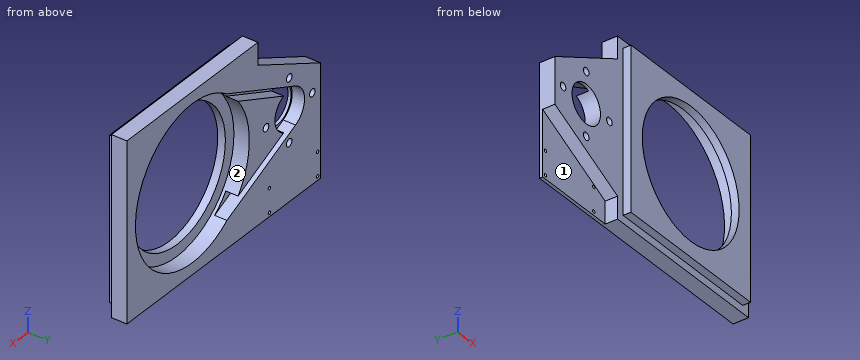
```python
from build123d import *

# Parameters (mm, degrees)
SKETCH1_W             = 105
SKETCH1_H             = 105
BOSS_EXTRUDE1_DEPTH   = 5
SKETCH2_W             = 115
SKETCH2_H             = 115
BOSS_EXTRUDE2_DEPTH   = 10
SKETCH3_R             = 42.5
CUT_EXTRUDE1_DEPTH    = 83.689177043
SKETCH4_R             = 50
CUT_EXTRUDE2_DEPTH    = 10
BOSS_EXTRUDE3_DEPTH   = 10
SKETCH6_R             = 12.5
CUT_EXTRUDE3_DEPTH    = 128.2301065
F_8_CLEARANCE_HOLE1_D = 4.9149
CUT_EXTRUDE4_DEPTH    = 8
SKETCH10_R            = 1
BOSS_EXTRUDE4_DEPTH   = 2


with BuildPart() as part:
    # Sketch1 → Boss-Extrude1 (new body)
    with BuildSketch(Plane(origin=(0, 0, 0), x_dir=(1, 0, 0), z_dir=(0, 1, 0))):
        Rectangle(SKETCH1_W, SKETCH1_H)
    extrude(amount=BOSS_EXTRUDE1_DEPTH)

    # Sketch2 → Boss-Extrude2 (add)
    with BuildSketch(Plane(origin=(0, 5, 0), x_dir=(1, 0, 0), z_dir=(0, 1, 0))):
        Rectangle(SKETCH2_W, SKETCH2_H)
    extrude(amount=BOSS_EXTRUDE2_DEPTH)

    # Sketch3 → Cut-Extrude1 (cut, through all)
    with BuildSketch(Plane(origin=(0, 15, 0), x_dir=(1, 0, 0), z_dir=(0, 1, 0))):
        with Locations(Location((0, 0, 0), (0, 0, 270))):
            Circle(SKETCH3_R)
    extrude(amount=-CUT_EXTRUDE1_DEPTH, mode=Mode.SUBTRACT)

    # Sketch4 → Cut-Extrude2 (cut)
    with BuildSketch(Plane(origin=(0, 15, 0), x_dir=(1, 0, 0), z_dir=(0, 1, 0))):
        with Locations(Location((0, 0, 0), (0, 0, 270))):
            Circle(SKETCH4_R)
    extrude(amount=-CUT_EXTRUDE2_DEPTH, mode=Mode.SUBTRACT)

    # Sketch5 → Boss-Extrude3 (add)
    with BuildSketch(Plane(origin=(0, 15, 0), x_dir=(1, 0, 0), z_dir=(0, 1, 0))):
        Polygon((-57.5, 43.090435246), (-57.5, -43.090435246), (-112.5, -15), (-112.5, 15), align=None)
    extrude(amount=-BOSS_EXTRUDE3_DEPTH)

    # Sketch6 → Cut-Extrude3 (cut, through all)
    with BuildSketch(Plane(origin=(0, 15, 0), x_dir=(1, 0, 0), z_dir=(0, 1, 0))):
        with Locations(Location((-85, 0, 0), (0, 0, 270))):
            Circle(SKETCH6_R)
    extrude(amount=-CUT_EXTRUDE3_DEPTH, mode=Mode.SUBTRACT)

    # #8 Clearance Hole1 (through all)
    with Locations(Plane(origin=(0, 5, 0), x_dir=(-1, 0, 0), z_dir=(0, -1, 0))):
        with Locations((64.64239577, 0), (85, -20.35760423), (105.35760423, 0), (85, 20.35760423)):
            Hole(F_8_CLEARANCE_HOLE1_D / 2)

    # Sketch9 → Cut-Extrude4 (cut)
    with BuildSketch(Plane(origin=(0, 15, 0), x_dir=(1, 0, 0), z_dir=(0, 1, 0))):
        with BuildLine():
            Line((-20.216911765, 44.360331138), (-90.598529412, 12.284399392))
            ThreePointArc((-90.598529412, 12.284399392), (-98.5, 0), (-90.598529412, -12.284399392))
            Line((-90.598529412, -12.284399392), (-20.216911765, -44.360331138))
            ThreePointArc((-20.216911765, -44.360331138), (-16.905258283, -43.122207068), (-18.143382353, -39.810553586))
            Line((-18.143382353, -39.810553586), (-88.525, -7.734621839))
            ThreePointArc((-88.525, -7.734621839), (-93.5, 0), (-88.525, 7.734621839))
            Line((-88.525, 7.734621839), (-18.143382353, 39.810553586))
            ThreePointArc((-18.143382353, 39.810553586), (-16.905258283, 43.122207068), (-20.216911765, 44.360331138))
        make_face()
    extrude(amount=-CUT_EXTRUDE4_DEPTH, mode=Mode.SUBTRACT)

    # Sketch10 → Boss-Extrude4 (add)
    with BuildSketch(Plane(origin=(0, 15, 0), x_dir=(1, 0, 0), z_dir=(0, 1, 0))):
        Polygon((-57.5, 57.5), (-112.5, 57.5), (-112.5, 15), (-57.5, 43.090435246), align=None)
        with Locations(Location((-67.6, 55, 0), (0, 0, 270))):
            Circle(SKETCH10_R, mode=Mode.SUBTRACT)
        with Locations(Location((-67.6, 39.6, 0), (0, 0, 270))):
            Circle(SKETCH10_R, mode=Mode.SUBTRACT)
        with Locations(Location((-110, 55, 0), (0, 0, 270))):
            Circle(SKETCH10_R, mode=Mode.SUBTRACT)
        with Locations(Location((-110, 39.6, 0), (0, 0, 270))):
            Circle(SKETCH10_R, mode=Mode.SUBTRACT)
    extrude(amount=-BOSS_EXTRUDE4_DEPTH)


solid = part.part
```
CAD build for the part. Positions are in the model's coordinates, mm. Face numbers are marked on the shaded views. Coordinates: 2 decimals unless noted, no trailing zeros. Order: outer loops, then holes, each group sorted by start corner. A loop starts at its lowest first (then second) coordinate and runs counter-clockwise, first axis right, second up.
(1) Saw through at C-C, the plane x = 0. Write the cut outline in (y, z).
Solution:
outline: (0, -52.5) - (5, -52.5) - (5, -57.5) - (15, -57.5) - (15, -50) - (5, -50) - (5, -42.5) - (0, -42.5) - close; (0, 42.5) - (5, 42.5) - (5, 50) - (15, 50) - (15, 57.5) - (5, 57.5) - (5, 52.5) - (0, 52.5) - close
(2) Mould opens along X. For the marked faces 1 and 2 say: released by +X, released by -X, zero draft, split by the parting line, or undercut.
Solution:
face 1: zero draft
face 2: undercut
(3) Drill centre lines: L1, parallel to X at y = 13.65, z = -55; L2, parallel to X at y = 1.9, z = 0; L3, parallel to Z at x = -85, y = 9. Where is each one in solid material? Low to high.
Solution:
L1: x = -112.5 to -111, -109 to -68.6, -66.6 to 57.5
L2: x = -52.5 to -42.5, 42.5 to 52.5
L3: z = -29.05 to -22.82, -17.9 to -14.84, 14.84 to 17.9, 22.82 to 29.05
(4) Saw through at D-D, the plane z = 27.5. Write the cut outline in (x, y).
Solution:
outline: (-88.03, 5) - (-52.5, 5) - (-52.5, 0) - (-32.4, 0) - (-32.4, 5) - (-41.76, 5) - (-41.76, 15) - (-45.16, 15) - (-45.16, 7) - (-57.21, 7) - (-57.21, 15) - (-88.03, 15) - close; (32.4, 0) - (52.5, 0) - (52.5, 5) - (57.5, 5) - (57.5, 15) - (41.76, 15) - (41.76, 5) - (32.4, 5) - close
(5) Saw through at A-A, the plane z = 0. Count the separate pieces of the cut face and the enclosed holes in it, and give its area (3 significant figures).
Solution:
separate pieces: 5
enclosed holes: 0
area: 444 mm2
(6) Pin check, flat tips, straight feed: pin 1 Ø1 at (x, z) = (-81.5, 22) entering from -Y; pin 2 Ø1.8 at (x, z) = (-67.6, -55) entering from +Y; pin 3 Ø1 at (x, y) = (-86.5, 5.5) entering from +Z; pin 4 Ø4 at (x, y) = (13.5, 1.5) entering from +Z. Stop position of each tip, or through.
Solution:
pin 1: stops at y = 5
pin 2: passes through
pin 3: stops at z = 28.53
pin 4: stops at z = 52.5
(7) Saw through at B-B, the plane y = 9.75. Write the cut outline in (x, z).
Solution:
outline: (-112.5, -15) - (-57.5, -43.09) - (-57.5, -57.5) - (57.5, -57.5) - (57.5, 57.5) - (-57.5, 57.5) - (-57.5, 43.09) - (-112.5, 15) - close; (-80.19, -11.54) - (-40.17, -29.77) arc R50 cw to (-40.17, 29.77) - (-80.19, 11.54) arc R12.5 cw to start; hole circle Ø4.91 at (-105.36, 0); hole (-90.6, -12.28) - (-30.33, -39.75) arc R50 ccw (long way) to (-30.33, 39.75) - (-90.6, 12.28) arc R13.5 ccw to start; hole circle Ø4.91 at (-85, -20.36); hole circle Ø4.91 at (-85, 20.36); hole circle Ø4.91 at (-64.64, 0)
